```python
from build123d import *

# Parameters (mm, degrees)
F0_R            = 20
F1_DEPTH        = 10
F3_DEPTH        = 8.5
F4_R            = 2
F5_DEPTH        = 10.001
F5_COPIES_COUNT = 6
F7_DEPTH        = 3.25
F7_COPIES_COUNT = 6
F8_R            = 5.08
F9_DEPTH        = 10.001
F10_R           = 9.144
F11_DEPTH       = 10.001
F13_DEPTH       = 8.128
F14_R           = 1.5875
F15_DEPTH       = 25.4


# Not quite as in the source:
# - a pattern or mirror of a feature is missing from the dataset's text; its kind, count and spacing are read off the source's solid


with BuildPart() as f1:
    # F0 (on Front) → F1 (new body)
    with BuildSketch(Plane.XZ):
        Circle(F0_R)
    extrude(amount=F1_DEPTH)

    # F2 (on face) → F3 (cut)
    with BuildSketch(Plane(origin=(0, 0, 0), x_dir=(-1, 0, 0), z_dir=(0, 1, 0))):
        Polygon((3.3197640478, 5.75), (-3.3197640478, 5.75), (-6.6395280957, 0), (-3.3197640478, -5.75), (3.3197640478, -5.75), (6.6395280957, 0), align=None)
    extrude(amount=-F3_DEPTH, mode=Mode.SUBTRACT)

    # F4 (on face) → F5 (cut, through all)
    with BuildSketch(Plane.XZ.offset(10)):
        with Locations((0, 15)):
            Circle(F4_R)
    f5 = extrude(amount=-F5_DEPTH, mode=Mode.SUBTRACT)

    # F5_copies: F5 ×6 about axis
    f5_copies_axis = Axis((0, 0, 0), (0, 1, 0))
    for i in range(1, F5_COPIES_COUNT):
        add(f5.rotate(f5_copies_axis, i * 360 / F5_COPIES_COUNT), mode=Mode.SUBTRACT)

    # F6 (on face) → F7 (cut)
    with BuildSketch(Plane.XZ.offset(10)):
        Polygon((2.375, 19.113620668), (-2.375, 19.113620668), (-4.75, 15), (-2.375, 10.886379332), (2.375, 10.886379332), (4.75, 15), align=None)
    f7 = extrude(amount=-F7_DEPTH, mode=Mode.SUBTRACT)

    # F7_copies: F7 ×6 about axis
    f7_copies_axis = Axis((0, 0, 0), (0, 1, 0))
    for i in range(1, F7_COPIES_COUNT):
        add(f7.rotate(f7_copies_axis, i * 360 / F7_COPIES_COUNT), mode=Mode.SUBTRACT)

    # F8 (on face) → F9 (cut, through all)
    with BuildSketch(Plane.XZ.offset(10)):
        Circle(F8_R)
    extrude(amount=-F9_DEPTH, mode=Mode.SUBTRACT)

    # F10 (on face) → F11 (cut, through all)
    with BuildSketch(Plane(origin=(0, 0, 0), x_dir=(-1, 0, 0), z_dir=(0, 1, 0))):
        Circle(F10_R)
    extrude(amount=-F11_DEPTH, mode=Mode.SUBTRACT)

    # F12 (on face) → F13 (cut)
    with BuildSketch(Plane(origin=(0, 0, 0), x_dir=(-1, 0, 0), z_dir=(0, 1, 0))):
        Polygon((9.2023301022, 13.0179032851), (6.6726698978, 14.4784032851), (-9.2023301022, -13.0179032851), (-6.6726698978, -14.4784032851), align=None)
    extrude(amount=-F13_DEPTH, mode=Mode.SUBTRACT)

    # F14 (on Right) → F15 (cut, symmetric)
    with BuildSketch(Plane.YZ):
        with Locations((-3.175, 0)):
            Circle(F14_R)
    extrude(amount=F15_DEPTH, both=True, mode=Mode.SUBTRACT)


solid = f1.part
```
Check sheet for the modelled part. Datum: model origin and axes. Units: mm. A direction names the side the tool comes from. Give positions to 0.01 mm unless a question says otherwise; leave off trailing zeros. Loops run counter-clockwise (first coordinate to the right, second up) from the corner with the lowest first, then second, coordinate; pieces in that order, holes last. Notation, with made-up numbers: (21, 75.5) - (63, 75.5) arc R23 ccw to (63, 103.5) - close; hole circle Ø6 at (-2.5, -40). An arc over 180 degrees is marked (long way). One line per question, with ' | ' between items. Start each with the question number.
1. Material ranges on line 1 along Z through (x, y) = (0, -0.25); line 2 along X through (y, z) = (-1.5, 6); line 3 along X through (y, z) = (-8, 0), recorded low to high. Write a range as [from, to].
2. Cross-section at C-C, the plane y = -1. Enter the section's corners in (x, z).
3. Set-up check for faces 1 (the cylindrical face through (-14.066, -3.422, 5.814)), 2 (the flat face through (-9.411, -8.398, 9.528)): record each of +Z, -Z, +X, -X, +Y, -Y from which the full face is reachable in a straight line by a thin tool's end or side.
4. Cross-section at A-A, the plane x = 1. Enter the section's corners in (y, z).
5. Draft check along Z on faces 3 (the flat face through (9, 0, -4)), 4 (the flat face through (7.466, -4.007, -10.011)). Enter one of: released by +Z, released by -Z, zero draft, split by the parting line, or undercut.
6. Gauge pin test, flat ends, axial feed: pin 1 Ø3.5 at (x, y) = (13.5, -8) entering from +Z; pin 2 Ø6 at (y, z) = (-2.5, 5.5) entering from -X; pin 3 Ø1.6 at (x, y) = (-0.5, -8.5) entering from -Z. Record the tip position at first contact, or that the pin passes through.
7. Cross-section at B-B, the plane z = 0. Enter the section's corners in (x, y).
8. Cross-section at D-D, the plane z = 4.5. Enter the section's corners in (x, y).
Check result:
1) line 1: z = [-20, -17], [-13, -9.14], [9.14, 13], [17, 20] | line 2: x = [-19.08, -14.31], [-11.67, -6.9], [6.9, 11.67], [14.31, 19.08] | line 3: x = [-20, -9.14], [9.14, 20]
2) outline: circle Ø40 at (0, 0); hole circle Ø4 at (-12.99, -7.5); hole circle Ø4 at (-12.99, 7.5); hole (-9.2, 13.02) - (-5.78, 7.09) arc R9.14 ccw to (3.25, -8.55) - (6.67, -14.48) - (9.2, -13.02) - (5.78, -7.09) arc R9.14 ccw to (-3.25, 8.55) - (-6.67, 14.48) - close; hole circle Ø4 at (0, -15); hole circle Ø4 at (0, 15); hole circle Ø4 at (12.99, -7.5); hole circle Ø4 at (12.99, 7.5)
3) face 1: +Y, -Y | face 2: -Y
4) outline: (-10, -19.97) - (0, -19.97) - (0, -16.73) - (-6.75, -16.73) - (-6.75, -19.11) - (-10, -19.11) - close; (-10, -10.89) - (-6.75, -10.89) - (-6.75, -13.27) - (0, -13.27) - (0, -9.09) - (-10, -9.09) - close; (-10, 9.09) - (0, 9.09) - (0, 13.27) - (-6.75, 13.27) - (-6.75, 10.89) - (-10, 10.89) - close; (-10, 19.11) - (-6.75, 19.11) - (-6.75, 16.73) - (0, 16.73) - (0, 19.97) - (-10, 19.97) - close
5) face 3: zero draft | face 4: undercut
6) pin 1: stops at z = 16.18 | pin 2: stops at x = -19.84 | pin 3: stops at z = -20
7) outline: (-20, -10) - (-9.14, -10) - (-9.14, -4.76) - (-20, -4.76) - close; (-20, -1.59) - (-9.14, -1.59) - (-9.14, 0) - (-20, 0) - close; (9.14, -10) - (20, -10) - (20, -4.76) - (9.14, -4.76) - close; (9.14, -1.59) - (20, -1.59) - (20, 0) - (9.14, 0) - close
8) outline: (-19.49, -10) - (-16.01, -10) - (-16.01, -6.75) - (-9.97, -6.75) - (-9.97, -10) - (-7.96, -10) - (-7.96, 0) - (-19.49, 0) - close; (7.96, -10) - (9.97, -10) - (9.97, -6.75) - (16.01, -6.75) - (16.01, -10) - (19.49, -10) - (19.49, 0) - (7.96, 0) - close
